from build123d import *

# Parameters (mm, degrees)
SKETCH1_R           = 7.934325
BOSS_EXTRUDE1_DEPTH = 47.625
SKETCH3_R           = 4.76885
CUT_EXTRUDE1_DEPTH  = 14.2875
SKETCH2_R           = 4.0259
CUT_EXTRUDE2_DEPTH  = 25.4
SKETCH5_R           = 4.352925
CUT_EXTRUDE3_DEPTH  = 3.175
CHAMFER1_SIZE       = 1.524


with BuildPart() as part:
    # Sketch1 → Boss-Extrude1 (new body)
    with BuildSketch(Plane.XY):
        Circle(SKETCH1_R)
    extrude(amount=-BOSS_EXTRUDE1_DEPTH)

    # Sketch3 → Cut-Extrude1 (cut, symmetric)
    with BuildSketch(Plane(origin=(0, 0, 0), x_dir=(1, 0, 0), z_dir=(0, 1, 0))):
        with Locations(Location((0, 23.8125, 0), (0, 0, 270))):
            Circle(SKETCH3_R)
    extrude(amount=CUT_EXTRUDE1_DEPTH, both=True, mode=Mode.SUBTRACT)

    # Sketch2 → Cut-Extrude2 (cut)
    with BuildSketch(Plane.XY):
        Circle(SKETCH2_R)
    extrude(amount=-CUT_EXTRUDE2_DEPTH, mode=Mode.SUBTRACT)

    # Sketch5 → Cut-Extrude3 (cut)
    with BuildSketch(Plane.XY):
        Circle(SKETCH5_R)
    extrude(amount=-CUT_EXTRUDE3_DEPTH, mode=Mode.SUBTRACT)

    # Chamfer1
    chamfer1_edges = [part.edges().sort_by_distance(p)[0] for p in [
        (-7.934325, 0, 0),
        (-7.934325, 0, -47.625),
    ]]
    chamfer(chamfer1_edges, length=CHAMFER1_SIZE)


solid = part.part
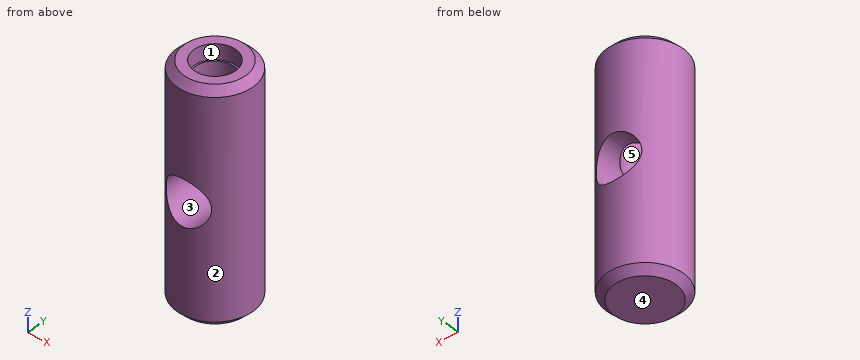
The listing builds one solid part. Answer for the finished solid, in the listing's coordinates (mm). Face numbers are marked on the shaded views. A direction names the side the tool comes from. Give positions to 0.01 mm unless a question says otherwise; leave off trailing zeros. Order: outer loops, then holes, each group sorted by start corner. A loop starts at its lowest first (then second) coordinate and runs counter-clockwise, first axis right, second up. Notation, with made-up numbers: (-40, 10.5) - (-27, 10.5) arc R27 cw to (-27, 47.5) - close; hole circle Ø1 at (23.25, -3.75). An arc over 180 degrees is marked (long way). One line per item, written item: value. Start each with the question number.
1) A cutting plane is placed at B-B on z = -5.5. Give the vertices of the cut face in (x, y), then the cut area to 3 significant figures.
2) Find the intervals of material crossed by L1, parallel to Z at x = -0.25, y = -7; L2, parallel to Z at x = -3.5, y = -2.5 (3 decimals); L3, parallel to Z at x = 0, y = 0 (3 decimals), in increasing order.
3) Given pin 1 Ø8 at (y, z) = (-5.5, -40) entering from -X; pin 2 Ø5 at (x, y) = (0, 0) entering from +Z; pin 3 Ø6 at (x, z) = (3.5, -5) entering from +Y, each flat-ended and moving along its own axis, determine where each tip first touches the part or whether it passes through.
4) A cutting plane is placed at C-C on z = -24.5. Give the vertices of the cut face in (x, y), then the cut area to 3 significant figures.
5) A tool of negligible diameter and unlimited length cuts with its end or side. For the marked faces 1 and 2, from which of +Z, -Z, +X, -X, +Y, -Y can it reach the whole face along a straight path? Write none if from no direction.
6) A cutting plane is placed at D-D on x = -3.25. State how many separate pieces and enclosed holes the cut face has, then the cut area to 3 significant figures.
7) The mould has two halves that part along Z. Classify the marked faces 3, 4 and 5: released by +Z, released by -Z, zero draft, split by the parting line, or undercut.
8) A cutting plane is placed at A-A on x = 0. Give the vertices of the cut face in (y, z) (3 decimals), then the cut area to 3 significant figures.
Answer sheet:
1. outline: circle Ø15.87 at (0, 0); hole circle Ø8.05 at (0, 0)
1. area: 147 mm2
2. L1: z = -47.03 to -28.57, -19.05 to -0.59
2. L2: z = -47.625 to -27.052, -20.573 to -3.175
2. L3: z = -47.625 to -28.581
3. pin 1: stops at x = -7.79
3. pin 2: stops at z = -27.87
3. pin 3: stops at y = 7.92
4. outline: (-4.72, -6.38) - (-4.72, 6.38) arc R7.93 ccw to start; (4.72, -6.38) arc R7.93 ccw to (4.72, 6.38) - close
4. area: 57.4 mm2
5. face 1: +Z
5. face 2: +Z, -Z
6. separate pieces: 3
6. enclosed holes: 0
6. area: 483 mm2
7. face 3: undercut
7. face 4: released by -Z
7. face 5: zero draft
8. outline: (-7.934, -46.101) - (-6.41, -47.625) - (6.41, -47.625) - (7.934, -46.101) - (7.934, -28.581) - (-7.934, -28.581) - close; (-7.934, -19.044) - (-4.026, -19.044) - (-4.026, -3.175) - (-4.353, -3.175) - (-4.353, 0) - (-6.41, 0) - (-7.934, -1.524) - close; (4.026, -19.044) - (7.934, -19.044) - (7.934, -1.524) - (6.41, 0) - (4.353, 0) - (4.353, -3.175) - (4.026, -3.175) - close
8. area: 444 mm2
